Geometry check sheet. Reference: the model listing, model coordinates, mm. Face numbers are marked on the shaded views. A direction names the side the tool comes from. Coordinates: 2 decimals unless noted, no trailing zeros. Write each loop counter-clockwise with the first axis right and the second up, starting at its lowest first coordinate (ties: lowest second). Pieces come first, ordered by that corner, then holes. Notation, with made-up numbers: (55.25, 26.5) -> (67.25, 26.5) arc R17 cw to (67.25, 58.5) -> close; hole circle Ø6 at (-25.5, 24.25). An arc over 180 degrees is marked (long way). Answer in a Markdown table with one row per item. Add a question column.
Q1. Section check A-A, the plane x = -15. Record the boundary of the cut face in (y, z), and give its area (3 significant figures).
Q2. Tool access check on the marked faces 4, 5 and 6. Record the directions out of +Z, -Z, +X, -X, +Y, -Y that give a thin tool (end or side, any length) a straight path to the whole face; none if there is none.
Q3. Section check C-C, the plane x = -32.93. Record the boundary of the cut face in (y, z), and give its area (3 significant figures).
Q4. Release check for a two-part mould opening along Z. For the marked faces 1, 2 and 3 record: pulls with the +Z half, pulls with the -Z half, needs draft (parallel to the pull), parting line crosses it, or undercut.
Q5. Section check D-D, the plane y = -21. Record the boundary of the cut face in (x, z), and give its area (3 significant figures).
Q6. Thickness scan on line 1 (Y direction, x = 32.93, z = 0.7); line 2 (Z direction, x = 31.5, y = -38); line 3 (X direction, y = -43.5, z = 4.5). Record the ranges inside material, lowest first.
Q7. Gauge pin test, flat ends, axial feed: P1, Ø1.5, axis at x = 15.5, z = 38, coming from the -Y side; P2, Ø3.5, axis at y = -7.5, z = 32, coming from the -X side; P3, Ø9.5, axis at x = 18, y = -9, coming from the +Z side; P4, Ø10, axis at x = -24, y = -25, coming from the -Z side. Record the tip position at first contact, or that the pin passes through.
Q8. Section check B-B, the plane z = 33.5. Record the boundary of the cut face in (x, y), and give its area (3 significant figures).
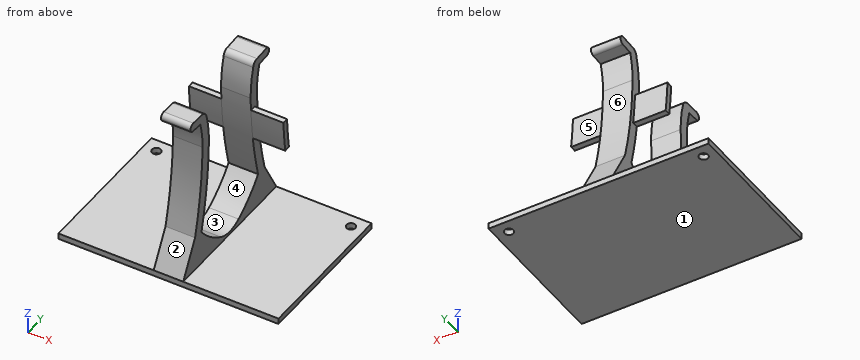
```python
from build123d import *
from build123d.topology import SkipClean

# Parameters (mm, degrees)
SKETCH1_R                = 1.5
BOSS_EXTRUDE1_DEPTH      = 2
BOSS_EXTRUDE2_DEPTH      = 5
BOSS_EXTRUDE2_DEPTH_BACK = 5
BOSS_EXTRUDE3_DEPTH      = 16
BOSS_EXTRUDE3_DEPTH_BACK = 16


with BuildPart() as part:
    # Sketch1 → Boss-Extrude1 (new body)
    with BuildSketch(Plane.XY):
        Polygon((32.93, 4.3095034), (-32.93, 4.3095034), (-37.2395034, 4.3095034), (-37.2395034, -46.928143845), (37.2395034, -46.928143845), (37.2395034, 4.3095034), align=None)
        with Locations((1.941, -42.566)):
            Circle(SKETCH1_R, mode=Mode.SUBTRACT)
        with Locations((-32.93, 0)):
            Circle(SKETCH1_R, mode=Mode.SUBTRACT)
        with Locations((32.93, 0)):
            Circle(SKETCH1_R, mode=Mode.SUBTRACT)
    extrude(amount=BOSS_EXTRUDE1_DEPTH)

    # Sketch2 → Boss-Extrude2 (add, two sides: drawn at the far end of the back side and taken through both)
    with BuildSketch(Plane(origin=(0, 0, 0), x_dir=(0, 0, -1), z_dir=(1, 0, 0)).offset(-BOSS_EXTRUDE2_DEPTH_BACK)):
        with BuildLine():
            Line((-13.827857709, -2.193698586), (-2, 4.3095034))
            Line((-2, 4.3095034), (0, 4.3095034))
            Line((0, 4.3095034), (0, -46.928143845))
            Line((0, -46.928143845), (-2, -46.928143845))
            Line((-2, -46.928143845), (-13.827857709, -40.424941859))
            ThreePointArc((-13.827857709, -40.424941859), (-29.0735826, -37.459870422), (-44.561553332, -36.299465883))
            ThreePointArc((-44.561553332, -36.299465883), (-49.270202349, -36.576792482), (-53.884612562, -37.55429133))
            Line((-53.884612562, -37.55429133), (-54.096567625, -41.562549641))
            ThreePointArc((-54.096567625, -41.562549641), (-55.64009753, -42.951035737), (-57.028583626, -41.407505832))
            Line((-57.028583626, -41.407505832), (-56.760743998, -36.342420783))
            ThreePointArc((-56.760743998, -36.342420783), (-56.091378633, -35.074236285), (-54.941875511, -34.216923926))
            ThreePointArc((-54.941875511, -34.216923926), (-49.777133912, -33.113502449), (-44.505153577, -32.799945311))
            ThreePointArc((-44.505153577, -32.799945311), (-28.861742138, -33.957189589), (-13.455691977, -36.908317202))
            ThreePointArc((-13.455691977, -36.908317202), (-8.292913419, -32.004111605), (-4.225812769, -26.159096012))
            ThreePointArc((-4.225812769, -26.159096012), (-2.971078619, -21.309320222), (-4.225812769, -16.459544433))
            ThreePointArc((-4.225812769, -16.459544433), (-8.292907204, -10.614536079), (-13.455676881, -5.710334914))
            ThreePointArc((-13.455676881, -5.710334914), (-28.861727042, -8.661462527), (-44.505138481, -9.818706805))
            ThreePointArc((-44.505138481, -9.818706805), (-49.777118817, -9.505149667), (-54.941860415, -8.40172819))
            ThreePointArc((-54.941860415, -8.40172819), (-56.291509436, -7.71567705), (-56.760743998, -6.276219662))
            Line((-56.760743998, -6.276219662), (-57.028583626, -1.211134613))
            ThreePointArc((-57.028583626, -1.211134613), (-55.64009753, 0.332395292), (-54.096567625, -1.056090804))
            Line((-54.096567625, -1.056090804), (-53.884612562, -5.064349115))
            ThreePointArc((-53.884612562, -5.064349115), (-49.270202349, -6.041847963), (-44.561553332, -6.319174562))
            ThreePointArc((-44.561553332, -6.319174562), (-29.0735826, -5.158770023), (-13.827857709, -2.193698586))
        make_face()
    extrude(amount=BOSS_EXTRUDE2_DEPTH + BOSS_EXTRUDE2_DEPTH_BACK)

    # Sketch5 → Boss-Extrude3 (add, two sides: drawn at the far end of the back side and taken through both)
    with SkipClean():  # the faces are left unmerged after this step: merging them gives an invalid solid
        with BuildSketch(Plane(origin=(0, 0, 0), x_dir=(0, 0, -1), z_dir=(1, 0, 0)).offset(-BOSS_EXTRUDE3_DEPTH_BACK)):
            with BuildLine():
                Line((-39.941860415, -7.665931491), (-39.941860415, -9.668427594))
                ThreePointArc((-39.941860415, -9.668427594), (-34.391490644, -9.278314981), (-28.861727042, -8.661462527))
                Line((-28.861727042, -8.661462527), (-28.874022965, -6.645436075))
                ThreePointArc((-28.874022965, -6.645436075), (-34.397354661, -7.270505974), (-39.941860415, -7.665931491))
            make_face()
        extrude(amount=BOSS_EXTRUDE3_DEPTH + BOSS_EXTRUDE3_DEPTH_BACK)


solid = part.part
```
Calculated:
| question | item | result |
|---|---|---|
| 1 | outline | (-46.93, 0) -> (4.31, 0) -> (4.31, 2) -> (-46.93, 2) -> close; (-9.67, 39.94) arc R135.98 ccw to (-8.66, 28.86) -> (-6.65, 28.87) arc R133.98 cw to (-7.67, 39.94) -> close |
| 1 | area | 125 mm² |
| 2 | face 4 | +X, -X |
| 2 | face 5 | +Z, +X, +Y |
| 2 | face 6 | +X, -X, +Y |
| 3 | outline | (-46.93, 0) -> (-1.5, 0) -> (-1.5, 2) -> (-46.93, 2) -> close; (1.5, 0) -> (4.31, 0) -> (4.31, 2) -> (1.5, 2) -> close |
| 3 | area | 96.5 mm² |
| 4 | face 1 | pulls with the -Z half |
| 4 | face 2 | undercut |
| 4 | face 3 | pulls with the +Z half |
| 5 | outline | (-37.24, 0) -> (37.24, 0) -> (37.24, 2) -> (5, 2) -> (5, 2.98) -> (-5, 2.98) -> (-5, 2) -> (-37.24, 2) -> close |
| 5 | area | 159 mm² |
| 6 | line 1 | y = -46.93 to -1.5, 1.5 to 4.31 |
| 6 | line 2 | z = 0 to 2 |
| 6 | line 3 | x = -5 to 5 |
| 7 | P1 | stops at y = -9.6 |
| 7 | P2 | stops at x = -16 |
| 7 | P3 | stops at z = 39.94 |
| 7 | P4 | stops at z = 0 |
| 8 | outline | (-16, -9.19) -> (16, -9.19) -> (16, -7.18) -> (5, -7.18) -> (5, -5.68) -> (-5, -5.68) -> (-5, -7.18) -> (-16, -7.18) -> close; (-5, -36.94) -> (5, -36.94) -> (5, -33.42) -> (-5, -33.42) -> close |
| 8 | area | 115 mm² |
